Build history of the part. All positions in model axes, mm. A direction names the side the tool comes from. Coordinates: 2 decimals unless noted, no trailing zeros. Order: outer loops, then holes, each group sorted by start corner. A loop starts at its lowest first (then second) coordinate and runs counter-clockwise, first axis right, second up. Notation, with made-up numbers: M 36,2 L 41,2 A25 ccw 41,17 Z; hole C 2.5,-11.75 d10. An arc over 180 degrees is marked long. Write item = value, one per line. Start each with the question number.
Q1. Pull direction X, two halves, no side cores. Call faces 3 (the face through (-1.08, -6.16, -4.88)), 4 (the face through (-2, -18, 3)), 5 (the face through (-2.539, -9.126, -1.947)): released by +X, released by -X, zero draft, split by the parting line, or undercut.
Q2. Band-saw the part on D-D on z = 3.5. Write the cut outline in (x, y).
Q3. Band-saw the part on B-B on x = 0. Write the cut outline in (y, z).
Q4. Band-saw the part on C-C on y = -15.75. Write the cut outline in (x, z).
Q5. 3-axis set-ups, long thin cutter, end or side, ignore diameter. For faces 1 (the face through (1, 0, -3.3)), 2 (the face through (-0.867, -15.212, -3.905)): which of +Z, -Z, +X, -X, +Y, -Y reach the whole face in a straight line?
Q6. Band-saw the part on A-A on z = 0. Write the cut outline in (x, y), plus the area to 3 significant figures.
Q7. Drill centre lines: probe 1 along Z at (x, y) = (0, -10.25); probe 2 along Y at (x, z) = (3.75, -2); probe 3 along Z at (x, y) = (-1.75, -16.5). Where is each one in solid material? Low to high.
Q8. Pin check, flat tips, straight feed: P1, Ø1.5, axis at y = -7, z = 2, coming from the +X side; P2, Ø2, axis at y = -2.5, z = -2.5, coming from the -X side. Stop position of each tip, or through.
```python
from build123d import *

# Parameters (mm, degrees)
F0_R     = 5
F1_DEPTH = 12.5
F2_R     = 4
F3_DEPTH = 5.5
F5_D     = 6.4


with BuildPart() as f1:
    # F0 (on Front) → F1 (new body)
    with BuildSketch(Plane.XZ):
        Circle(F0_R)
    extrude(amount=F1_DEPTH)

    # F2 (on face) → F3 (join)
    with BuildSketch(Plane.XZ.offset(12.5)):
        Circle(F2_R)
    extrude(amount=F3_DEPTH)

    # F5 (through all)
    with Locations(Plane(origin=(0, 0, 0), x_dir=(-1, 0, 0), z_dir=(0, 1, 0))):
        with Locations((0, 0)):
            Hole(F5_D / 2)


solid = f1.part
```
Recorded:
q1.face_3 = split by the parting line
q1.face_4 = zero draft
q1.face_5 = undercut
q2.outline = M -3.57,-12.5 L -1.94,-12.5 L -1.94,-18 L 1.94,-18 L 1.94,-12.5 L 3.57,-12.5 L 3.57,0 L -3.57,0 Z
q3.outline = M -18,-4 L -12.5,-4 L -12.5,-5 L 0,-5 L 0,-3.2 L -18,-3.2 Z; M -18,3.2 L 0,3.2 L 0,5 L -12.5,5 L -12.5,4 L -18,4 Z
q4.outline = C 0,0 d8; hole C 0,0 d6.4
q5.face_1 = +Z, -Z, +X, -X, +Y
q5.face_2 = -Y
q6.outline = M -5,-12.5 L -4,-12.5 L -4,-18 L -3.2,-18 L -3.2,0 L -5,0 Z; M 3.2,-18 L 4,-18 L 4,-12.5 L 5,-12.5 L 5,0 L 3.2,0 Z
q6.area = 53.8 mm2
q7.probe_1 = -5 to -3.2, 3.2 to 5
q7.probe_2 = -12.5 to 0
q7.probe_3 = -3.6 to -2.68, 2.68 to 3.6
q8.P1 = 4.84
q8.P2 = -4.77
